```python
from build123d import *

# Parameters (mm, degrees)
BOSS_EXTRU_1_DEPTH      = 6.35
ESQUISSE3_R             = 36.322
ENL_V_MAT_EXTRU_2_DEPTH = 173.855351378
ENL_V_MAT_EXTRU_5_DEPTH = 6.35
ESQUISSE7_R             = 1.75
ENL_V_MAT_EXTRU_6_DEPTH = 6.35


with BuildPart() as part:
    # Esquisse1 → Boss.-Extru.1 (new body)
    with BuildSketch(Plane(origin=(0, 0, 0), x_dir=(1, 0, 0), z_dir=(0, 1, 0))):
        Polygon((-101.6, 139.7), (-101.6, 127), (-74.6125, 127), (-31.75, 0), (31.75, 0), (74.6125, 127), (101.6, 127), (101.6, 139.7), align=None)
    extrude(amount=BOSS_EXTRU_1_DEPTH)

    # Esquisse3 → Enlèv. mat.-Extru.2 (cut, through all)
    with BuildSketch(Plane(origin=(0, 6.35, 0), x_dir=(1, 0, 0), z_dir=(0, 1, 0))):
        with Locations(Location((0, 63.5, 0), (0, 0, 270))):
            Circle(ESQUISSE3_R)
    extrude(amount=-ENL_V_MAT_EXTRU_2_DEPTH, mode=Mode.SUBTRACT)

    # Esquisse6 → Enlèv. mat.-Extru.5 (cut)
    with BuildSketch(Plane(origin=(0, 6.35, 0), x_dir=(1, 0, 0), z_dir=(0, 1, 0))):
        with BuildLine():
            Line((-36.322, 63.5), (-36.322, 139.7))
            Line((-36.322, 139.7), (36.322, 139.7))
            Line((36.322, 139.7), (36.322, 63.5))
            ThreePointArc((36.322, 63.5), (0, 99.822), (-36.322, 63.5))
        make_face()
    extrude(amount=-ENL_V_MAT_EXTRU_5_DEPTH, mode=Mode.SUBTRACT)

    # Esquisse7 → Enlèv. mat.-Extru.6 (cut)
    with BuildSketch(Plane(origin=(0, 6.35, 0), x_dir=(1, 0, 0), z_dir=(0, 1, 0))):
        with Locations(Location((0, 20.701, 0), (0, 0, 270))):
            Circle(ESQUISSE7_R)
        with Locations(Location((42.54026093, 58.801, 0), (0, 0, 270))):
            Circle(ESQUISSE7_R)
        with Locations(Location((-42.54026093, 58.801, 0), (0, 0, 270))):
            Circle(ESQUISSE7_R)
    extrude(amount=-ENL_V_MAT_EXTRU_6_DEPTH, mode=Mode.SUBTRACT)


solid = part.part
```
Input: part model. Units: mm. Frame: model coordinates. A direction names the side the tool comes from. Give positions to 0.01 mm unless a question says otherwise; leave off trailing zeros. Write each loop counter-clockwise with the first axis right and the second up, starting at its lowest first coordinate (ties: lowest second). Pieces come first, ordered by that corner, then holes. Notation, with made-up numbers: (72.25, 44) - (98.25, 44) arc R27 cw to (98.25, 71) - close; hole circle Ø3 at (19.25, 43.5). An arc over 180 degrees is marked (long way). Write item = value, one per line. Start each with the question number.
1) Reachability of faces 1 (the face through (-88, 3, -127)), 2 (the face through (69, 3, -139.7)), 3 (the face through (88, 3, -127)) from +Z, -Z, +X, -X, +Y, -Y: full face, straight path, thin tool, end or side. Return the list, or none.
2) Pin query (flat end, axial travel): pin 1 (3 mm diameter, centred on x = 0, z = -20.701, fed in from +Y); pin 2 (3 mm diameter, centred on y = 4.5, z = -117, fed in from +X). Return the tip coordinate at first contact, or that it passes through.
3) Material intervals for L1, parallel to X at y = 3.75, z = -131; L2, parallel to X at y = 5.25, z = -109; L3, parallel to Z at x = 77, y = 4.75, sorted ascending. Write a range as [from, to].
4) Cut plane A-A (z = -47.5). Return loops of the section in (x, y), and give its area (3 significant figures).
5) Cut plane B-B (y = 2.75). Return loops of the section in (x, z).
6) Draft query along X for faces 4 (the face through (-101.6, 3, -133)), 5 (the face through (36.322, 3, -102)), 6 (the face through (-36.322, 3, -101)), 7 (the face through (-69, 3, -139.7)). Return one class per face: pulls with the +X half, pulls with the -X half, needs draft (parallel to the pull), parting line crosses it, or undercut.
7) Cut plane C-C (z = -69). Return loops of the section in (x, y), and give its area (3 significant figures).
8) Cut plane D-D (x = -12). Return loops of the section in (y, z), and give its area (3 significant figures).
Answers follow:
q1.face_1 = +Z, -X, +Y, -Y
q1.face_2 = -Z, +X, -X, +Y, -Y
q1.face_3 = +Z, +X, +Y, -Y
q2.pin_1 = through
q2.pin_2 = 71.74
q3.L1 = [-101.6, -36.32], [36.32, 101.6]
q3.L2 = [-68.54, -36.32], [36.32, 68.54]
q3.L3 = [-139.7, -127]
q4.outline = (-47.78, 0) - (-32.61, 0) - (-32.61, 6.35) - (-47.78, 6.35) - close; (32.61, 0) - (47.78, 0) - (47.78, 6.35) - (32.61, 6.35) - close
q4.area = 193 mm^2
q5.outline = (-101.6, -139.7) - (-36.32, -139.7) - (-36.32, -63.5) arc R36.32 cw to (36.32, -63.5) - (36.32, -139.7) - (101.6, -139.7) - (101.6, -127) - (74.61, -127) - (31.75, 0) - (-31.75, 0) - (-74.61, -127) - (-101.6, -127) - close; hole circle Ø3.5 at (-42.54, -58.8); hole circle Ø3.5 at (0, -20.7); hole circle Ø3.5 at (42.54, -58.8)
q6.face_4 = pulls with the -X half
q6.face_5 = undercut
q6.face_6 = undercut
q6.face_7 = needs draft
q7.outline = (-55.04, 0) - (-36.32, 0) - (-36.32, 6.35) - (-55.04, 6.35) - close; (36.32, 0) - (55.04, 0) - (55.04, 6.35) - (36.32, 6.35) - close
q7.area = 238 mm^2
q8.outline = (0, -29.22) - (6.35, -29.22) - (6.35, 0) - (0, 0) - close
q8.area = 186 mm^2
